Geometry check sheet. Reference: the model listing, model coordinates, mm. Face numbers are marked on the shaded views. A direction names the side the tool comes from. Coordinates: 2 decimals unless noted, no trailing zeros. Write each loop counter-clockwise with the first axis right and the second up, starting at its lowest first coordinate (ties: lowest second). Pieces come first, ordered by that corner, then holes. Notation, with made-up numbers: (65.5, 1.5) -> (86.5, 1.5) arc R15 cw to (86.5, 5.5) -> close; hole circle Ø10 at (31.25, 41.25). An arc over 180 degrees is marked (long way). Put each result on its own line as item: value. Start each with the question number.
from build123d import *

# Parameters (mm, degrees)
F0_W     = 22
F0_H     = 35
F1_DEPTH = 6.3
F2_R     = 6.7597979746
F3_R     = 2.65
F5_D     = 2.7
F5_DEPTH = 15
F5_TIP   = 0.8111618357


with BuildPart() as f1:
    # F0 (on Top) → F1 (new body)
    with BuildSketch(Plane.XY):
        Rectangle(F0_W, F0_H)
    extrude(amount=F1_DEPTH)

    # F2
    f2_edges = [f1.edges().sort_by_distance(p)[0] for p in [
        (-11, -17.5, 3.15),
        (11, -17.5, 3.15),
    ]]
    fillet(f2_edges, radius=F2_R)

    # F3
    f3_edges = [f1.edges().sort_by_distance(p)[0] for p in [
        (-11, 3.379899, 6.3),
        (-11, 3.379899, 0),
    ]]
    fillet(f3_edges, radius=F3_R)

    # F5
    with Locations(Plane(origin=(0, 17.5, 0), x_dir=(-1, 0, 0), z_dir=(0, 1, 0))):
        with Locations((0, 3.15)):
            Hole(F5_D / 2, depth=F5_DEPTH)
            with Locations((0, 0, -(F5_DEPTH + F5_TIP / 2))):  # 118° drill point
                Cone(0, F5_D / 2, F5_TIP, mode=Mode.SUBTRACT)


solid = f1.part
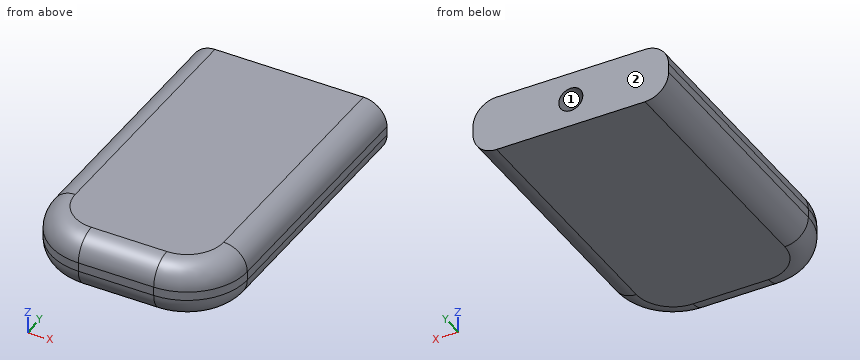
Item 1: Scan lines: line 1 along X through (y, z) = (10.5, 3); line 2 along Z through (x, y) = (0, 12.75); line 3 along Y through (x, z) = (-4.5, 2.75) (3 decimals). Record each from-to range of solid material in increasing order. Write a range as [from, to].
Item 2: Access from +Z, -Z, +X, -X, +Y, -Y to the whole of each face (thin tool, end or side, straight path). Record for the marked faces 1 and 2.
Item 3: Section check A-A, the plane y = -2. Enter the section's corners in (x, z).
Item 4: Go/stop test with flat-tipped pins: P1, Ø1, axis at x = 5, z = 3.5, coming from the -Y side (3 decimals); P2, Ø2, axis at y = -9, z = 4.5, coming from the -X side. Record where each tip stops, or that it passes through.
Item 5: Section check B-B, the plane z = 1. Enter the section's corners in (x, y), and give its area (3 significant figures).
From the geometry:
1. line 1: [-11, -1.34], [1.34, 11]
1. line 2: [0, 1.8], [4.5, 6.3]
1. line 3: [-17.495, 17.5]
2. face 1: +Y
2. face 2: +Z, -Z, +X, -X, +Y
3. outline: (-11, 2.65) arc R2.65 ccw to (-8.35, 0) -> (8.35, 0) arc R2.65 ccw to (11, 2.65) -> (11, 3.65) arc R2.65 ccw to (8.35, 6.3) -> (-8.35, 6.3) arc R2.65 ccw to (-11, 3.65) -> close
4. P1: y = -17.495
4. P2: x = -11
5. outline: (-10.42, -10.74) arc R6.18 ccw to (-4.24, -16.92) -> (4.24, -16.92) arc R6.18 ccw to (10.42, -10.74) -> (10.42, 17.5) -> (-10.42, 17.5) -> close
5. area: 701 mm²
